Design review of the part built by this model. Coordinates are the model's own, in mm. A direction names the side the tool comes from. Give positions to 0.01 mm unless a question says otherwise; leave off trailing zeros. Loops run counter-clockwise (first coordinate to the right, second up) from the corner with the lowest first, then second, coordinate; pieces in that order, holes last. Notation, with made-up numbers: (0, 12.25) -> (5, 12.25) arc R13 ccw to (5, 37.25) -> close; hole circle Ø8 at (79.5, 67). An arc over 180 degrees is marked (long way). Use CSV: the item, a comma, the result in double quotes. Start each with the question number.
Item 1: Wall thickness on line 1 along X through (y, z) = (5.25, -7) (1 decimal); line 2 along X through (y, z) = (-3.25, -3); line 3 along Y through (x, z) = (117, -0.25): over which ranges is each line inside the solid? List them lowest first. Write a range as from..to.
Item 2: Clearance check with flat-ended pins moving along their axes: pin 1 (1.5 mm diameter, centred on x = 98, y = -1.5, fed in from -Z); pin 2 (1.1 mm diameter, centred on x = 129, y = 4, fed in from -Z); pin 3 (7 mm diameter, centred on x = 27.5, z = -1, fed in from +Y). State where each tip first meets the part, or that it passes through.
Item 3: The part is to be moulded in two halves that separate along X. For faces 4 (the face through (138.112, 0, 0)), 5 (the face through (48.53, -1.72, 7.75)), 6 (the face through (3.96, -1.72, 7.75)), say which applies: +X half, -X half, draft (parallel to the pull), parting line (faces both ways), or undercut.
Item 4: We need section A-A (x = 90). State the section outline as (y, z) points (1 decimal), plus the area to 3 significant figures.
Item 5: For faces 1 (the face through (3.175, 2, -8)), 2 (the face through (136.5, -3.78, 2.9)), 3 (the face through (25, 6.35, 0)), list the 3-axis set-ups (+Z, -Z, +X, -X, +Y, -Y) from which the entire face can be reached by the end or side of a thin tool; tool diameter is ignored.
from build123d import *

# Parameters (mm, degrees)
CUT_EXTRUDE1_DEPTH = 3.175
CUT_EXTRUDE2_DEPTH = 1.5875


with BuildPart() as part:
    # Sketch2 → Revolve1 (revolve)
    with BuildSketch(Plane.XY):
        Polygon((0, 0), (138.1125, 0), (138.1125, 4.7625), (134.9375, 4.7625), (134.9375, 3.175), (133.35, 3.175), (133.35, 4.7625), (122.8725, 4.7625), (122.8725, 6.35), (116.5225, 6.35), (116.5225, 7.9375), (53.34, 7.9375), (53.34, 6.35), (51.7525, 6.35), (51.7525, 7.9375), (45.4025, 7.9375), (45.4025, 9.525), (4.7625, 9.525), (4.7625, 7.9375), (3.175, 7.9375), (3.175, 9.525), (0, 9.525), align=None)
    revolve(axis=Axis((0, 0, 0), (-1, 0, 0)))

    # Sketch3 → Cut-Extrude1 (cut)
    with BuildSketch(Plane(origin=(0, 9.525, 0), x_dir=(1, 0, 0), z_dir=(0, 1, 0))):
        with BuildLine():
            Line((15.5575, 3.175), (34.6075, 3.175))
            ThreePointArc((34.6075, 3.175), (37.7825, 0), (34.6075, -3.175))
            Line((34.6075, -3.175), (15.5575, -3.175))
            ThreePointArc((15.5575, -3.175), (12.3825, 0), (15.5575, 3.175))
        make_face()
    extrude(amount=-CUT_EXTRUDE1_DEPTH, mode=Mode.SUBTRACT)

    # Sketch4 → Cut-Extrude2 (cut)
    with BuildSketch(Plane(origin=(0, 4.7625, 0), x_dir=(1, 0, 0), z_dir=(0, 1, 0))):
        with BuildLine():
            Line((125.73, 1.5875), (130.4925, 1.5875))
            ThreePointArc((130.4925, 1.5875), (132.08, 0), (130.4925, -1.5875))
            Line((130.4925, -1.5875), (125.73, -1.5875))
            ThreePointArc((125.73, -1.5875), (124.1425, 0), (125.73, 1.5875))
        make_face()
    extrude(amount=-CUT_EXTRUDE2_DEPTH, mode=Mode.SUBTRACT)


solid = part.part
Results found:
1,line 1,"0..3.2, 4.8..45.4"
1,line 2,"0..133.35, 134.94..138.11"
1,line 3,"-6.35..6.35"
2,pin 1,"z = -7.9"
2,pin 2,"z = -3.28"
2,pin 3,"y = 8.98"
3,face 4,"+X half"
3,face 5,"draft"
3,face 6,"undercut"
4,outline,"circle Ø15.9 at (0, 0)"
4,area,"198 mm²"
5,face 1,"none"
5,face 2,"+X"
5,face 3,"+Y"
